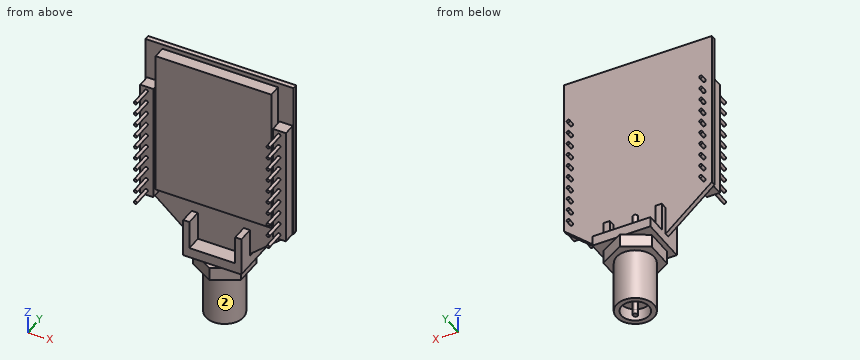
from build123d import *

# Parameters (mm, degrees)
BASE_PCB_DEPTH                      = 0.7874
SKETCH2_R                           = 0.254
HEADER_HOLE_DEPTH                   = 1.7874
F_2MM_HEADER_PATTERN_COUNT          = 10
F_2MM_HEADER_PATTERN_PITCH          = 2
F_2MM_HEADER_PATTERN_COUNT_DIR2     = 2
F_2MM_HEADER_PATTERN_PITCH_DIR2     = 21.844
SKETCH3_W                           = 19.05
SKETCH3_H                           = 24.13
WIRELESS_MODULE_DEPTH               = 2.032
HEADER_START                        = -6.096
SKETCH12_R                          = 0.254
HEADER_PIN_DEPTH                    = 7.112
F_2MM_HEADER_PIN_PATTERN_COUNT      = 10
F_2MM_HEADER_PIN_PATTERN_PITCH      = 2
F_2MM_HEADER_PIN_PATTERN_COUNT_DIR2 = 2
F_2MM_HEADER_PIN_PATTERN_PITCH_DIR2 = 21.844
SKETCH13_W                          = 2.159
SKETCH13_H                          = 19.558
HEADER_BOSS_DEPTH                   = 2.032
HEADER_BOSS_PATTERN_COUNT           = 2
HEADER_BOSS_PATTERN_PITCH           = 21.844
SKETCH4_W                           = 9.5758
SKETCH4_H                           = 7.874
SMA_BASE_DEPTH                      = 1.651
SKETCH5_W                           = 1.016
SKETCH5_H                           = 2.54
SMA_PRONGS_BOTTOM_DEPTH             = 4.699
SKETCH6_W                           = 1.016
SKETCH6_H                           = 1.143
SMA_PRONGS_TOP_DEPTH                = 4.699
SKETCH7_R                           = 0.381
SMA_CENTER_PIN_DEPTH                = 4.699
SMA_CENTER_PIN_DEPTH_BACK           = 13.208
SMA_NUT_DEPTH                       = 2.159
SKETCH10_R                          = 3.1115
RPSMA_BARREL_DEPTH                  = 8.636
SKETCH11_R                          = 2.286
SKETCH11_R_2                        = 0.381
CUT_EXTRUDE4_DEPTH                  = 2.032


with BuildPart() as part:
    # Sketch1 → Base PCB (new body)
    with BuildSketch(Plane(origin=(0, 0, 0), x_dir=(1, 0, 0), z_dir=(0, 1, 0))):
        Polygon((0, 26.416), (7.62, 33.02), (16.764, 33.02), (24.384, 26.416), (24.384, 0), (0, 0), align=None)
    extrude(amount=BASE_PCB_DEPTH)

    # Sketch2 → Header Hole (cut, through all)
    with BuildSketch(Plane(origin=(0, 0.7874, 0), x_dir=(1, 0, 0), z_dir=(0, 1, 0))):
        with Locations((1.27, 7.62)):
            Circle(SKETCH2_R)
    header_hole = extrude(amount=-HEADER_HOLE_DEPTH, mode=Mode.SUBTRACT)

    # 2mm Header pattern: Header Hole 10 × 2
    with Locations(*[(j * F_2MM_HEADER_PATTERN_PITCH_DIR2, 0, -i * F_2MM_HEADER_PATTERN_PITCH) for i in range(F_2MM_HEADER_PATTERN_COUNT) for j in range(F_2MM_HEADER_PATTERN_COUNT_DIR2) if (i, j) != (0, 0)]):
        add(header_hole, mode=Mode.SUBTRACT)

    # Sketch3 → Wireless Module (add)
    with BuildSketch(Plane.XZ):
        with Locations((12.319, -12.827)):
            Rectangle(SKETCH3_W, SKETCH3_H)
    extrude(amount=WIRELESS_MODULE_DEPTH)

    # Sketch12 → Header Pin (add)
    with BuildSketch(Plane(origin=(0, 0.7874, 0), x_dir=(1, 0, 0), z_dir=(0, 1, 0)).offset(HEADER_START)):
        with Locations((1.27, 7.62)):
            Circle(SKETCH12_R)
    header_pin = extrude(amount=HEADER_PIN_DEPTH)

    # 2mm Header Pin pattern: Header Pin 10 × 2
    with Locations(*[(j * F_2MM_HEADER_PIN_PATTERN_PITCH_DIR2, 0, -i * F_2MM_HEADER_PIN_PATTERN_PITCH) for i in range(F_2MM_HEADER_PIN_PATTERN_COUNT) for j in range(F_2MM_HEADER_PIN_PATTERN_COUNT_DIR2) if (i, j) != (0, 0)]):
        add(header_pin)

    # Sketch13 → Header Boss (add)
    with BuildSketch(Plane.XZ):
        with Locations((23.1775, -16.637)):
            Rectangle(SKETCH13_W, SKETCH13_H)
    header_boss = extrude(amount=HEADER_BOSS_DEPTH)

    # Header Boss pattern: Header Boss ×2
    with Locations(*[(-i * HEADER_BOSS_PATTERN_PITCH, 0, 0) for i in range(1, HEADER_BOSS_PATTERN_COUNT)]):
        add(header_boss)

    # Sketch4 → SMA Base (add)
    with BuildSketch(Plane(origin=(0, 0, -33.02), x_dir=(-1, 0, 0), z_dir=(0, 0, -1))):
        with Locations((-12.4079, 1.397)):
            Rectangle(SKETCH4_W, SKETCH4_H)
    extrude(amount=SMA_BASE_DEPTH)

    # Sketch5 → SMA Prongs-bottom (add)
    with BuildSketch(Plane.XY.offset(-33.02)):
        with Locations((8.128, -1.27)):
            Rectangle(SKETCH5_W, SKETCH5_H)
        with Locations((16.6878, -1.27)):
            Rectangle(SKETCH5_W, SKETCH5_H)
    extrude(amount=SMA_PRONGS_BOTTOM_DEPTH)

    # Sketch6 → SMA Prongs-top (add)
    with BuildSketch(Plane.XY.offset(-33.02)):
        with Locations((8.128, 1.3589)):
            Rectangle(SKETCH6_W, SKETCH6_H)
        with Locations((16.6878, 1.3589)):
            Rectangle(SKETCH6_W, SKETCH6_H)
    extrude(amount=SMA_PRONGS_TOP_DEPTH)

    # Sketch7 → SMA Center Pin (add, two sides)
    with BuildSketch(Plane.XY.offset(-33.02)) as sma_center_pin_sk:
        with Locations((12.4206, 1.143)):
            Circle(SKETCH7_R)
    extrude(amount=SMA_CENTER_PIN_DEPTH)
    extrude(sma_center_pin_sk.sketch, amount=-SMA_CENTER_PIN_DEPTH_BACK)

    # Sketch9 → SMA Nut (add)
    with BuildSketch(Plane(origin=(0, 0, -34.671), x_dir=(-1, 0, 0), z_dir=(0, 0, -1))):
        Polygon((-12.4206, 5.747714807), (-16.4084, 3.445357403), (-16.4084, -1.159357403), (-12.4206, -3.461714807), (-8.4328, -1.159357403), (-8.4328, 3.445357403), align=None)
    extrude(amount=SMA_NUT_DEPTH)

    # Sketch10 → RPSMA Barrel (add)
    with BuildSketch(Plane(origin=(0, 0, -36.83), x_dir=(-1, 0, 0), z_dir=(0, 0, -1))):
        with Locations((-12.4206, 1.143)):
            Circle(SKETCH10_R)
    extrude(amount=RPSMA_BARREL_DEPTH)

    # Sketch11 → Cut-Extrude4 (cut)
    with BuildSketch(Plane(origin=(0, 0, -45.466), x_dir=(-1, 0, 0), z_dir=(0, 0, -1))):
        with Locations((-12.4206, 1.143)):
            Circle(SKETCH11_R)
        with Locations((-12.4206, 1.143)):
            Circle(SKETCH11_R_2, mode=Mode.SUBTRACT)
    extrude(amount=-CUT_EXTRUDE4_DEPTH, mode=Mode.SUBTRACT)


solid = part.part
Work out the finished part from the listing and answer in its coordinate system (mm). Face numbers are marked on the shaded views. Give positions to 0.01 mm unless a question says otherwise; leave off trailing zeros. Write each loop counter-clockwise with the first axis right and the second up, starting at its lowest first coordinate (ties: lowest second). Pieces come first, ordered by that corner, then holes. Notation, with made-up numbers: (43.5, -23.5) - (51.5, -23.5) arc R29 ccw to (51.5, 10.5) - close; hole circle Ø4 at (46.5, -35). An arc over 180 degrees is marked (long way). One line per item, written item: value. Start each with the question number.
1. Consider probe 1 along X at (y, z) = (-1, -16.5); probe 2 along Z at (x, y) = (15.5, -2); probe 3 along Z at (x, y) = (9, 2.5). Determine where each line is inside the solid, lowest interval first.
2. Find section C-C (z = -34). Write down the section's boundary in (x, y), then the cut area to 3 significant figures.
3. Find section B-B (x = 5.25). Write down the section's boundary in (y, z), then the cut area to 3 significant figures.
4. For a pull along X with two mould halves and no side action, classify the marked faces 1 and 2 as +X half, -X half, draft (parallel to the pull), parting line (faces both ways), or undercut.
5. Find section A-A (y = -4.5). State how many separate pieces and enclosed holes the cut face has, then the cut area to 3 significant figures.
6. Find section D-D (x = 19). Write down the section's boundary in (y, z), then the cut area to 3 significant figures.
7. Given pin 1 (1.9 mm diameter, centred on x = 14, z = -31, fed in from -Y); pin 2 (1.6 mm diameter, centred on x = 12, y = -1.5, fed in from -Z); pin 3 (8 mm diameter, centred on x = 6.5, z = -39.5, fed in from -Y); pin 4 (3 mm diameter, centred on y = 4.5, z = -24.5, fed in from -X), each flat-ended and moving along its own axis, determine where each tip first touches the part or whether it passes through.
Geometry results:
1. probe 1: 0.25 to 2.41, 2.79 to 21.84, 22.1 to 24.26
1. probe 2: -34.67 to -33.02, -24.89 to -0.76
1. probe 3: -36.83 to -33.02
2. outline: (7.62, -2.54) - (17.2, -2.54) - (17.2, 5.33) - (7.62, 5.33) - close
2. area: 75.4 mm2
3. outline: (-2.03, -24.89) - (0, -24.89) - (0, -30.97) - (0.79, -30.97) - (0.79, 0) - (0, 0) - (0, -0.76) - (-2.03, -0.76) - close
3. area: 73.4 mm2
4. face 1: undercut
4. face 2: parting line
5. separate pieces: 20
5. enclosed holes: 0
5. area: 4.05 mm2
6. outline: (-2.03, -24.89) - (0, -24.89) - (0, -31.08) - (0.79, -31.08) - (0.79, 0) - (0, 0) - (0, -0.76) - (-2.03, -0.76) - close
6. area: 73.5 mm2
7. pin 1: y = 0
7. pin 2: z = -45.47
7. pin 3: y = -1.76
7. pin 4: through
